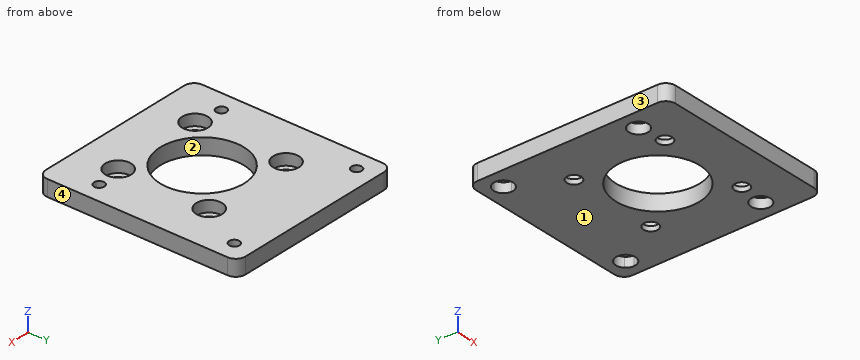
from build123d import *

# Parameters (mm, degrees)
SKETCH1_R           = 1.6
SKETCH1_R_2         = 13
SKETCH1_R_3         = 2.25
BOSS_EXTRUDE1_DEPTH = 5
SKETCH1_5_R         = 1.6
SKETCH1_5_R_2       = 3
CUT_EXTRUDE1_DEPTH  = 3
SKETCH2_R           = 4
CUT_EXTRUDE2_DEPTH  = 3.5


with BuildPart() as part:
    # Sketch1 → Boss-Extrude1 (new body)
    with BuildSketch(Plane.XY):
        with BuildLine():
            Line((-192.025912834, 67.472903007), (-141.025912834, 67.472903007))
            ThreePointArc((-141.025912834, 67.472903007), (-138.90459249, 66.59422335), (-138.025912834, 64.472903007))
            Line((-138.025912834, 64.472903007), (-138.025912834, 8.472903007))
            ThreePointArc((-138.025912834, 8.472903007), (-138.90459249, 6.351582663), (-141.025912834, 5.472903007))
            Line((-141.025912834, 5.472903007), (-192.025912834, 5.472903007))
            ThreePointArc((-192.025912834, 5.472903007), (-194.147233178, 6.351582663), (-195.025912834, 8.472903007))
            Line((-195.025912834, 8.472903007), (-195.025912834, 64.472903007))
            ThreePointArc((-195.025912834, 64.472903007), (-194.147233178, 66.59422335), (-192.025912834, 67.472903007))
        make_face()
        with Locations((-189.025912834, 61.472903007)):
            Circle(SKETCH1_R, mode=Mode.SUBTRACT)
        with Locations((-189.025912834, 19.472903007)):
            Circle(SKETCH1_R, mode=Mode.SUBTRACT)
        with Locations((-144.025912834, 19.472903007)):
            Circle(SKETCH1_R, mode=Mode.SUBTRACT)
        with Locations((-144.025912834, 61.472903007)):
            Circle(SKETCH1_R, mode=Mode.SUBTRACT)
        with Locations((-166.525912834, 32.472903007)):
            Circle(SKETCH1_R_2, mode=Mode.SUBTRACT)
        with Locations((-180.668048458, 18.330767383)):
            Circle(SKETCH1_R_3, mode=Mode.SUBTRACT)
        with Locations((-180.668048458, 46.61503863)):
            Circle(SKETCH1_R_3, mode=Mode.SUBTRACT)
        with Locations((-152.38377721, 46.61503863)):
            Circle(SKETCH1_R_3, mode=Mode.SUBTRACT)
        with Locations((-152.38377721, 18.330767383)):
            Circle(SKETCH1_R_3, mode=Mode.SUBTRACT)
    extrude(amount=BOSS_EXTRUDE1_DEPTH)

    # Sketch1_5 → Cut-Extrude1 (cut)
    # profile 1 of 4: a face of its own
    with BuildSketch(Plane.XY):
        with BuildLine():
            ThreePointArc((-186.025912834, 61.472903007), (-186.90459249, 63.59422335), (-189.025912834, 64.472903007))
            ThreePointArc((-189.025912834, 64.472903007), (-191.147233178, 63.59422335), (-192.025912834, 61.472903007))
            ThreePointArc((-192.025912834, 61.472903007), (-189.025912834, 58.472903007), (-186.025912834, 61.472903007))
        make_face()
        with Locations((-189.025912834, 61.472903007)):
            Circle(SKETCH1_5_R, mode=Mode.SUBTRACT)
    # profile 2 of 4: a face of its own
    with BuildSketch(Plane.XY):
        with BuildLine():
            ThreePointArc((-141.931336581, 63.620634442), (-146.79030506, 60.307512248), (-141.025912834, 61.472903007))
            ThreePointArc((-141.025912834, 61.472903007), (-141.261520608, 62.638293765), (-141.931336581, 63.620634442))
        make_face()
        with Locations((-144.025912834, 61.472903007)):
            Circle(SKETCH1_5_R, mode=Mode.SUBTRACT)
    # profile 3 of 4: a face of its own
    with BuildSketch(Plane.XY):
        with Locations((-144.025912834, 19.472903007)):
            Circle(SKETCH1_5_R_2)
        with Locations((-144.025912834, 19.472903007)):
            Circle(SKETCH1_5_R, mode=Mode.SUBTRACT)
    # profile 4 of 4: a face of its own
    with BuildSketch(Plane.XY):
        with Locations((-189.025912834, 19.472903007)):
            Circle(SKETCH1_5_R_2)
        with Locations((-189.025912834, 19.472903007)):
            Circle(SKETCH1_5_R, mode=Mode.SUBTRACT)
    extrude(amount=CUT_EXTRUDE1_DEPTH, mode=Mode.SUBTRACT)

    # Sketch2 → Cut-Extrude2 (cut)
    with BuildSketch(Plane.XY.offset(5)):
        with Locations((-180.668048458, 46.61503863)):
            Circle(SKETCH2_R)
        with Locations((-152.38377721, 46.61503863)):
            Circle(SKETCH2_R)
        with Locations((-152.38377721, 18.330767383)):
            Circle(SKETCH2_R)
        with Locations((-180.668048458, 18.330767383)):
            Circle(SKETCH2_R)
    extrude(amount=-CUT_EXTRUDE2_DEPTH, mode=Mode.SUBTRACT)


solid = part.part
Work out the finished part from the listing and answer in its coordinate system (mm). Face numbers are marked on the shaded views. Coordinates: 2 decimals unless noted, no trailing zeros. Loops run counter-clockwise (first coordinate to the right, second up) from the corner with the lowest first, then second, coordinate; pieces in that order, holes last. Notation, with made-up numbers: (-5, 6.25) -> (46, 6.25) arc R24 ccw to (46, 28.25) -> close; hole circle Ø6 at (11, -4.5). An arc over 180 degrees is marked (long way). Answer as CSV lines item,"result".
1) The part is cut by section D-D (z = 2.25). State how many separate pieces and enclosed holes the cut face has, and give its area (3 significant figures).
A:
separate pieces,"1"
enclosed holes,"9"
area,"2,680 mm²"
2) Flat-ended cylindrical pins translate along their axes: pin 1 (1.9 mm diameter, centred on x = -144.03, y = 19.47, fed in from -Z); pin 2 (5.5 mm diameter, centred on x = -189.03, y = 19.47, fed in from -Z). Find the tip coordinate at first contact, or state that the pin passes through.
A:
pin 1,"passes through"
pin 2,"stops at z = 3"
3) The part is cut by section C-C (x = -144). Give the vertices of the cut face in (y, z), and give its area (3 significant figures).
A:
outline,"(5.47, 0) -> (16.47, 0) -> (16.47, 3) -> (17.87, 3) -> (17.87, 5) -> (5.47, 5) -> close; (21.07, 3) -> (22.47, 3) -> (22.47, 0) -> (58.47, 0) -> (58.47, 3) -> (59.87, 3) -> (59.87, 5) -> (21.07, 5) -> close; (63.07, 3) -> (64.47, 3) -> (64.47, 0) -> (67.47, 0) -> (67.47, 5) -> (63.07, 5) -> close"
area,"261 mm²"
4) The part is cut by section A-A (y = 26). Give the vertices of the cut face in (x, z).
A:
outline,"(-195.03, 0) -> (-177.8, 0) -> (-177.8, 5) -> (-195.03, 5) -> close; (-155.25, 0) -> (-138.03, 0) -> (-138.03, 5) -> (-155.25, 5) -> close"
5) For a pull along X with two mould halves and no side action, classify the marked faces 1, 2, 3 and 4 as released by +X, released by -X, zero draft, split by the parting line, or undercut.
A:
face 1,"zero draft"
face 2,"undercut"
face 3,"released by -X"
face 4,"released by +X"
6) The part is cut by section B-B (x = -177.5). Give the vertices of the cut face in (y, z).
A:
outline,"(5.47, 0) -> (25.5, 0) -> (25.5, 5) -> (20.77, 5) -> (20.77, 1.5) -> (15.89, 1.5) -> (15.89, 5) -> (5.47, 5) -> close; (39.44, 0) -> (67.47, 0) -> (67.47, 5) -> (49.06, 5) -> (49.06, 1.5) -> (44.17, 1.5) -> (44.17, 5) -> (39.44, 5) -> close"
7) Straight lines are drawn through the part: probe 1 along Y at (x, z) = (-144, 1.95); probe 2 along X at (y, z) = (17, 2.2); probe 3 along Y at (x, z) = (-189.5, 2.45). For each, find the intervals that lie inside material, in ascending order.
A:
probe 1,"y = 5.47 to 16.47, 22.47 to 58.47, 64.47 to 67.47"
probe 2,"x = -195.03 to -190.72, -187.33 to -184.44, -176.9 to -156.16, -148.61 to -145.72, -142.33 to -138.03"
probe 3,"y = 5.47 to 16.51, 22.44 to 58.51, 64.44 to 67.47"
